from build123d import *

# Parameters (mm, degrees)
CUT_EXTRUDE1_DEPTH = 15
CUT_EXTRUDE2_DEPTH = 97.309063486


with BuildPart() as part:
    # Sketch2 → Revolve1 (revolve)
    with BuildSketch(Plane.XY, mode=Mode.PRIVATE) as revolve1_sk:
        Polygon((0, 0), (-4, 0), (-4, -5), (-6, -5), (-6, -12.5), (-6.75, -12.5), (-6.75, -15.25), (-14.9815, -15.25), (-14.9815, -48.11), (-16.8815, -48.11), (-16.8815, -51.11), (-8.25, -51.11), (-8.25, -53.61), (-7.5, -53.61), (-7.5, -58.61), (-6, -58.61), (-6, -92.535), (0, -92.535), align=None)
    revolve(revolve1_sk.sketch.rotate(Axis((0, 40.033449689, 0), (0, -1, 0)), 270), axis=Axis((0, 40.033449689, 0), (0, -1, 0)))

    # Sketch3 → Cut-Extrude1 (cut)
    with BuildSketch(Plane.XZ.offset(92.535)):
        with BuildLine():
            Line((-2, 5.656854249), (-2, 3.8))
            Line((-2, 3.8), (2, 3.8))
            Line((2, 3.8), (2, 5.656854249))
            ThreePointArc((2, 5.656854249), (0, 6), (-2, 5.656854249))
        make_face()
    extrude(amount=-CUT_EXTRUDE1_DEPTH, mode=Mode.SUBTRACT)

    # Sketch4 → Cut-Extrude2 (cut, through all)
    with BuildSketch(Plane.XY.offset(3.8)):
        with BuildLine():
            Line((-2, -77.535), (-2, -74.535))
            ThreePointArc((-2, -74.535), (0, -72.535), (2, -74.535))
            Line((2, -74.535), (2, -77.535))
            Line((2, -77.535), (2, -92.535))
            Line((2, -92.535), (-2, -92.535))
            Line((-2, -92.535), (-2, -77.535))
        make_face()
    extrude(amount=CUT_EXTRUDE2_DEPTH, mode=Mode.SUBTRACT)


solid = part.part
Input: part model. Units: mm. Frame: model coordinates. A direction names the side the tool comes from. Give positions to 0.01 mm unless a question says otherwise; leave off trailing zeros. Write each loop counter-clockwise with the first axis right and the second up, starting at its lowest first coordinate (ties: lowest second). Pieces come first, ordered by that corner, then holes. Notation, with made-up numbers: M 16.25,14.25 L 66.25,14.25 A18 cw 66.25,39.25 Z; hole C -4.75,-3.75 d10. An arc over 180 degrees is marked long. Use one line per item in the form item = value.
1. Cut plane D-D on x = -9.5. Return loops of the section in (y, z), and give its area (3 significant figures).
Outcome:
outline = M -51.11,-13.95 L -48.11,-13.95 L -48.11,-11.58 L -15.25,-11.58 L -15.25,11.58 L -48.11,11.58 L -48.11,13.95 L -51.11,13.95 Z
area = 845 mm²
2. Cut plane C-C on y = -34. Return loops of the section in (x, z), and give its area (3 significant figures).
Outcome:
outline = C 0,0 d29.96
area = 705 mm²
3. Ray query, L1, parallel to X at y = -56, z = -4.5; L2, parallel to Y at x = -2, z = -9.5; L3, parallel to Y at x = 5.5, z = 5. Return the intervals inside material, ascending.
Outcome:
L1 = -6 to 6
L2 = -51.11 to -15.25
L3 = -58.61 to -15.25
4. Reachability of faces 4 (the face through (0, 0, 0)), 5 (the face through (7, -53.61, 4)), 6 (the face through (0, -92.535, 0)), 7 (the face through (3.905, -2.535, -0.867)), 8 (the face through (-2, -84, 5)) from +Z, -Z, +X, -X, +Y, -Y: full face, straight path, thin tool, end or side. Return the list, or none.
Outcome:
face_4 = +Z, -Z, +X, -X, +Y
face_5 = -Y
face_6 = +Z, -Z, +X, -X, -Y
face_7 = +Y
face_8 = +Z, -Y
5. Mould query, pull axis X, two halves, no side actions, for faces 1 (the face through (3.92, -5, 1.42)), 2 (the face through (10.27, -49.63, -13.4)), 3 (the face through (-0.044, -72.535, 4.885)). Classes: released by +X, released by -X, zero draft, split by the parting line, or undercut.
Outcome:
face_1 = zero draft
face_2 = split by the parting line
face_3 = undercut
6. First-contact query: P1, Ø4.5, axis at x = 0, y = -79, coming from the +Z side; P2, Ø5, axis at x = -3, y = -29.5, coming from the +Z side; P3, Ø1.5, axis at y = -80, z = 4.5, coming from the -X side; P4, Ø3.5, axis at x = -1, z = -3, coming from the +Y side. Flat tips, straight axial feed; report the tip coordinate or a pass-through.
Outcome:
P1 = 5.66
P2 = 14.97
P3 = -4.68
P4 = 0
